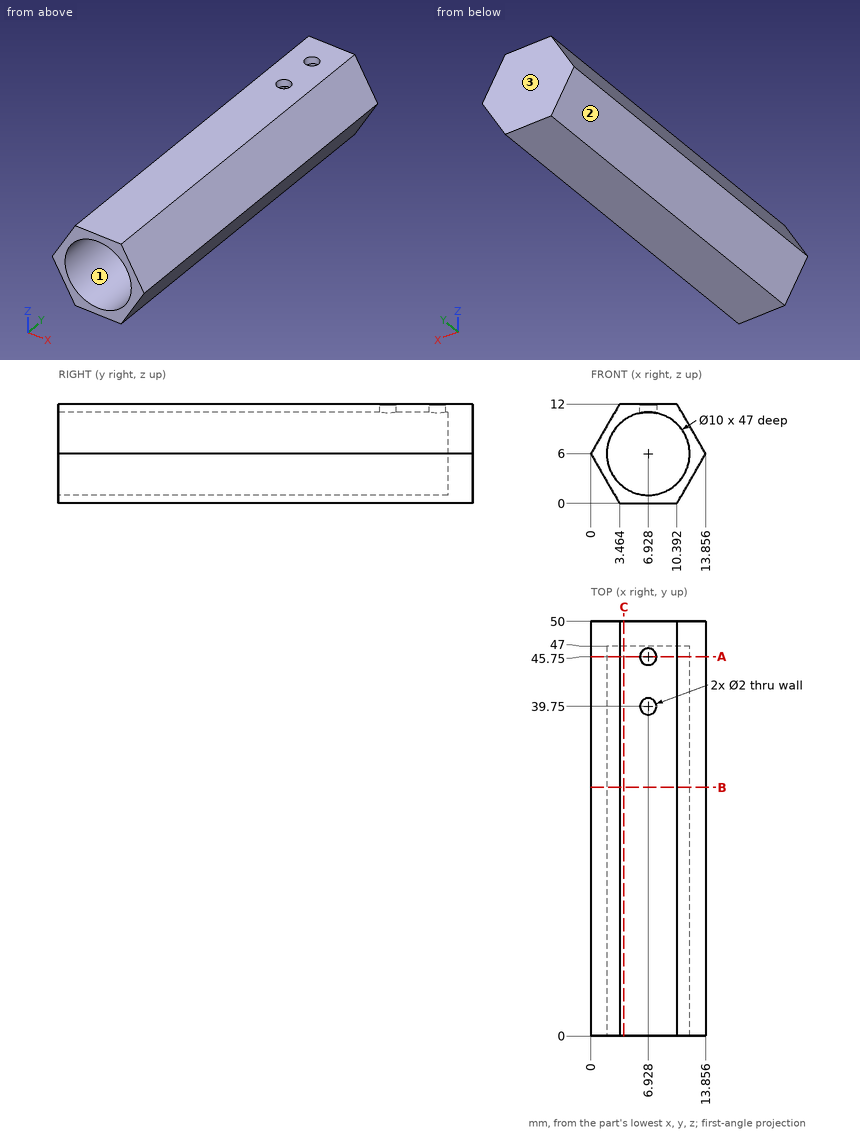
Verification items for this drawing (mm, ordinates from the low corner). Round coordinates to 2 decimals unless told otherwise and drop trailing zeros. Order: outer loops, then holes, each group sorted by start corner. A loop starts at its lowest first (then second) coordinate and runs counter-clockwise, first axis right, second up. Notation, with made-up numbers: (16, 4.5) - (28, 4.5) arc R19 ccw to (28, 14.5) - close; hole circle Ø8 at (34.5, 1.5). An arc over 180 degrees is marked (long way). Answer as CSV lines item,"result". Start each with the question number.
1) Section check C-C (x = 4). Record the cut outline in (y, z).
2) Scan lines: probe 1 along Z at (x, y) = (7, 8.5); probe 2 along Y at (x, z) = (5.25, 3); probe 3 along Z at (x, y) = (10.5, 35) (1 decimal). Record each from-to range of solid material in increasing order.
3) Section check A-A (y = 45.75). Record the cut outline in (x, z).
4) Draft check along X on the marked faces 1, 2 and 3. Enter one of: +X half, -X half, draft (parallel to the pull), parting line (faces both ways), or undercut.
5) Section check B-B (y = 30). Record the cut outline in (x, z).
6) Depth check by flat-ended pin: pin 1 (1 mm diameter, centred on y = 6.5, z = 2.5, fed in from -X); pin 2 (1 mm diameter, centred on x = 3, z = 8, fed in from -Y); pin 3 (3 mm diameter, centred on y = 33, z = 9.5, fed in from +X). Enter the tip coordinate at first touch or a pass-through.
Determined:
1,outline,"(0, 0) - (50, 0) - (50, 12) - (0, 12) - (0, 10.05) - (47, 10.05) - (47, 1.95) - (0, 1.95) - close"
2,probe 1,"0 to 1, 11 to 12"
2,probe 2,"47 to 50"
2,probe 3,"0.2 to 2.5, 9.5 to 11.8"
3,outline,"(0, 6) - (3.46, 0) - (10.39, 0) - (13.86, 6) - (10.39, 12) - (7.93, 12) - (7.93, 10.9) arc R5 cw (long way) to (5.93, 10.9) - (5.93, 12) - (3.46, 12) - close"
4,face 1,"undercut"
4,face 2,"-X half"
4,face 3,"draft"
5,outline,"(0, 6) - (3.46, 0) - (10.39, 0) - (13.86, 6) - (10.39, 12) - (3.46, 12) - close; hole circle Ø10 at (6.93, 6)"
6,pin 1,"x = 1.73"
6,pin 2,"y = 47"
6,pin 3,"x = 12.7"
